CAD build for the part. Positions are in the model's coordinates, mm. A direction names the side the tool comes from. Round coordinates to 2 decimals unless told otherwise and drop trailing zeros. Write each loop counter-clockwise with the first axis right and the second up, starting at its lowest first coordinate (ties: lowest second). Pieces come first, ordered by that corner, then holes. Notation, with made-up numbers: (-27, 42.25) - (6, 42.25) arc R13 ccw to (6, 55.25) - close; hole circle Ø9 at (68.25, -9). An arc over 180 degrees is marked (long way). Use one line per item in the form item = value. Start each with the question number.
Item 1: Tool access for faces 1 (the cylindrical face through (-30.325, 48.536, 2.873)), 2 (the flat face through (0, -41.8, 2)), 3 (the flat face through (35, -1, 2)): list every direction of +Z, -Z, +X, -X, +Y, -Y with a clear straight run to the whole face (end or side of a thin tool).
Item 2: Band-saw the part on A-A, the plane y = 0. List the corners of the cut face in (x, z), and give its area (3 significant figures).
Item 3: Pin check, flat tips, straight feed: pin 1 (0.8 mm diameter, centred on x = 0, z = 4.5, fed in from +Y); pin 2 (2 mm diameter, centred on x = -25.5, y = -35.5, fed in from +Z); pin 3 (1.5 mm diameter, centred on x = 30, y = 50.5, fed in from +Z); pin 4 (17 mm diameter, centred on x = 10.5, y = -12.5, fed in from +Z). Stop position of each tip, or through.
Item 4: Band-saw the part on B-B, the plane x = -18. List the corners of the cut face in (y, z).
Item 5: Band-saw the part on D-D, the plane y = 37. List the corners of the cut face in (x, z), and give its area (3 significant figures).
Item 6: Pull direction Y, two halves, no side cores. Call faces 4 (the cylindrical face through (34, 53, 2)), 5 (the cylindrical face through (29.675, 48.536, 2.873)), 6 (the cylindrical face through (33, -54, 2)): +Y half, -Y half, draft (parallel to the pull), parting line (faces both ways), or undercut.
Item 7: Drill centre lines: L1, parallel to Y at x = 30, z = 3.4; L2, parallel to X at y = 10.5, z = 0.75; L3, parallel to Y at x = -12.5, z = 3.75. Where is each one in solid material? Low to high.
Item 8: Band-saw the part on C-C, the plane z = 2.95. List the corners of the cut face in (x, y), and give its area (3 significant figures).
from build123d import *

# Parameters (mm, degrees)
F0_R     = 1.5
F1_DEPTH = 1
F2_DEPTH = 3.8
F3_DEPTH = 4.8


with BuildPart() as f1:
    # F0 (on Top) → F1 (new body)
    with BuildSketch(Plane.XY):
        with Locations((-30, 50)):
            Circle(F0_R)
    extrude(amount=F1_DEPTH)



with BuildPart() as f1b:
    # F0 (on Top) → F1, piece 2 (new body)
    with BuildSketch(Plane.XY):
        with Locations((30, 50)):
            Circle(F0_R)
    extrude(amount=F1_DEPTH)


with BuildPart() as f1c:
    # F0 (on Top) → F1, piece 3 (new body)
    with BuildSketch(Plane.XY):
        with Locations((30, 0)):
            Circle(F0_R)
    extrude(amount=F1_DEPTH)


with BuildPart() as f1d:
    # F0 (on Top) → F1, piece 4 (new body)
    with BuildSketch(Plane.XY):
        with Locations((30, -50)):
            Circle(F0_R)
    extrude(amount=F1_DEPTH)


with BuildPart() as f1e:
    # F0 (on Top) → F1, piece 5 (new body)
    with BuildSketch(Plane.XY):
        with Locations((-30, -50)):
            Circle(F0_R)
    extrude(amount=F1_DEPTH)


with BuildPart() as f1f:
    # F0 (on Top) → F1, piece 6 (new body)
    with BuildSketch(Plane.XY):
        with Locations((-30, 0)):
            Circle(F0_R)
    extrude(amount=F1_DEPTH)


with BuildPart() as f2:
    # F0 (on Top) → F2 (new body)
    with BuildSketch(Plane.XY):
        with BuildLine():
            Line((27.05, 42.8), (27.05, 55))
            Line((27.05, 55), (-27.05, 55))
            Line((-27.05, 55), (-27.05, 42.8))
            Line((-27.05, 42.8), (-27.05, -38.0607364771))
            ThreePointArc((-27.05, -38.0607364771), (-26.1012649001, -37.4476793164), (-25, -37.196376726))
            Line((-25, -37.196376726), (-25, 41.8))
            Line((-25, 41.8), (25, 41.8))
            Line((25, 41.8), (25, -37.2939372294))
            ThreePointArc((25, -37.2939372294), (26.0922729799, -37.5033114474), (27.05, -38.0686934251))
            Line((27.05, -38.0686934251), (27.05, 42.8))
        make_face()
        with BuildLine():
            ThreePointArc((-25, -37.196376726), (-26.1012649001, -37.4476793164), (-27.05, -38.0607364771))
            Line((-27.05, -38.0607364771), (-27.05, -42.8))
            Line((-27.05, -42.8), (-22.6016124349, -42.8))
            ThreePointArc((-22.6016124349, -42.8), (-22.1959427347, -42.3341702613), (-21.8857373462, -41.8))
            Line((-21.8857373462, -41.8), (-25, -41.8))
            Line((-25, -41.8), (-25, -37.196376726))
        make_face()
        with BuildLine():
            Line((-27.05, -42.8), (-27.05, -38.0607364771))
            ThreePointArc((-27.05, -38.0607364771), (-27.208254731, -42.6665921352), (-22.6016124349, -42.8))
            Line((-22.6016124349, -42.8), (-27.05, -42.8))
        make_face()
        with BuildLine():
            ThreePointArc((-21.8857373462, -41.8), (-22.1959427347, -42.3341702613), (-22.6016124349, -42.8))
            Line((-22.6016124349, -42.8), (22.6044172499, -42.8))
            ThreePointArc((22.6044172499, -42.8), (22.2287912639, -42.3305781393), (21.9460571083, -41.8))
            Line((21.9460571083, -41.8), (-21.8857373462, -41.8))
        make_face()
        with BuildLine():
            Line((27.05, -42.8), (27.05, -38.0686934251))
            ThreePointArc((27.05, -38.0686934251), (26.0922729799, -37.5033114474), (25, -37.2939372294))
            Line((25, -37.2939372294), (25, -41.8))
            Line((25, -41.8), (21.9460571083, -41.8))
            ThreePointArc((21.9460571083, -41.8), (22.2287912639, -42.3305781393), (22.6044172499, -42.8))
            Line((22.6044172499, -42.8), (27.05, -42.8))
        make_face()
        with BuildLine():
            ThreePointArc((28.1933165581, -40.5434428822), (27.8936742641, -39.1803987131), (27.05, -38.0686934251))
            Line((27.05, -38.0686934251), (27.05, -42.8))
            Line((27.05, -42.8), (22.6044172499, -42.8))
            ThreePointArc((22.6044172499, -42.8), (26.1600904172, -43.557072152), (28.1933165581, -40.5434428822))
        make_face()
    extrude(amount=F2_DEPTH)


with BuildPart() as f1_1:
    add(f1.part)

    add(f1b.part)  # F3 merges F1b

    add(f1c.part)  # F3 merges F1c

    add(f1d.part)  # F3 merges F1d

    add(f1e.part)  # F3 merges F1e

    add(f1f.part)  # F3 merges F1f

    add(f2.part)  # F3 merges F2
    # F0 (on Top) → F3 (join)
    with BuildSketch(Plane.XY):
        with BuildLine():
            ThreePointArc((35, 50), (33.5355339059, 53.5355339059), (30, 55))
            Line((30, 55), (27.05, 55))
            Line((27.05, 55), (27.05, 42.8))
            Line((27.05, 42.8), (27.05, -38.0686934251))
            ThreePointArc((27.05, -38.0686934251), (27.8936742641, -39.1803987131), (28.1933165581, -40.5434428822))
            ThreePointArc((28.1933165581, -40.5434428822), (26.1600904172, -43.557072152), (22.6044172499, -42.8))
            Line((22.6044172499, -42.8), (-22.6016124349, -42.8))
            ThreePointArc((-22.6016124349, -42.8), (-27.208254731, -42.6665921352), (-27.05, -38.0607364771))
            Line((-27.05, -38.0607364771), (-27.05, 42.8))
            Line((-27.05, 42.8), (-27.05, 55))
            Line((-27.05, 55), (-30, 55))
            ThreePointArc((-30, 55), (-33.5355339059, 53.5355339059), (-35, 50))
            Line((-35, 50), (-35, -50))
            ThreePointArc((-35, -50), (-33.5355339059, -53.5355339059), (-30, -55))
            Line((-30, -55), (30, -55))
            ThreePointArc((30, -55), (33.5355339059, -53.5355339059), (35, -50))
            Line((35, -50), (35, 50))
        make_face()
        with Locations((-30, -50)):
            Circle(F0_R, mode=Mode.SUBTRACT)
        with Locations((30, -50)):
            Circle(F0_R, mode=Mode.SUBTRACT)
        with Locations((-30, 0)):
            Circle(F0_R, mode=Mode.SUBTRACT)
        with Locations((-30, 50)):
            Circle(F0_R, mode=Mode.SUBTRACT)
        with Locations((30, 0)):
            Circle(F0_R, mode=Mode.SUBTRACT)
        with Locations((30, 50)):
            Circle(F0_R, mode=Mode.SUBTRACT)
    extrude(amount=F3_DEPTH)


solid = f1_1.part
Determined:
q1.face_1 = +Z
q1.face_2 = +Z, -Z
q1.face_3 = +Z, -Z, +X, +Y, -Y
q2.outline = (-35, 0) - (-25, 0) - (-25, 3.8) - (-27.05, 3.8) - (-27.05, 4.8) - (-28.5, 4.8) - (-28.5, 1) - (-31.5, 1) - (-31.5, 4.8) - (-35, 4.8) - close; (25, 0) - (35, 0) - (35, 4.8) - (31.5, 4.8) - (31.5, 1) - (28.5, 1) - (28.5, 4.8) - (27.05, 4.8) - (27.05, 3.8) - (25, 3.8) - close
q2.area = 69.1 mm²
q3.pin_1 = -42.8
q3.pin_2 = 3.8
q3.pin_3 = 1
q3.pin_4 = through
q4.outline = (-55, 0) - (-41.8, 0) - (-41.8, 3.8) - (-42.8, 3.8) - (-42.8, 4.8) - (-55, 4.8) - close; (41.8, 0) - (55, 0) - (55, 3.8) - (41.8, 3.8) - close
q5.outline = (-35, 0) - (-25, 0) - (-25, 3.8) - (-27.05, 3.8) - (-27.05, 4.8) - (-35, 4.8) - close; (25, 0) - (35, 0) - (35, 4.8) - (27.05, 4.8) - (27.05, 3.8) - (25, 3.8) - close
q5.area = 91.9 mm²
q6.face_4 = +Y half
q6.face_5 = undercut
q6.face_6 = -Y half
q7.L1 = -55 to -51.5, -48.5 to -1.5, 1.5 to 48.5, 51.5 to 55
q7.L2 = -35 to -25, 25 to 35
q7.L3 = -55 to -41.8, 41.8 to 55
q8.outline = (-35, -50) arc R5 ccw to (-30, -55) - (30, -55) arc R5 ccw to (35, -50) - (35, 50) arc R5 ccw to (30, 55) - (-30, 55) arc R5 ccw to (-35, 50) - close; hole circle Ø3 at (-30, -50); hole circle Ø3 at (-30, 0); hole circle Ø3 at (-30, 50); hole (-25, -41.8) - (25, -41.8) - (25, 41.8) - (-25, 41.8) - close; hole circle Ø3 at (30, -50); hole circle Ø3 at (30, 0); hole circle Ø3 at (30, 50)
q8.area = 3,460 mm²
